Input: part model. Units: mm. Frame: model coordinates. Face numbers are marked on the shaded views. A direction names the side the tool comes from. Coordinates: 2 decimals unless noted, no trailing zeros. Loops run counter-clockwise (first coordinate to the right, second up) from the corner with the lowest first, then second, coordinate; pieces in that order, holes last. Notation, with made-up numbers: (68.5, 32.25) -> (91.5, 32.25) arc R25 ccw to (91.5, 46.25) -> close; hole circle Ø3 at (20.25, -31.5). An arc over 180 degrees is marked (long way). Put each result on its own line as item: value. Start each with the question number.
1) Contact query for flat-ended pins moving along their axis: P1, Ø10.5, axis at x = 27, z = 6, coming from the -Y side; P2, Ø3, axis at y = -16.5, z = 3, coming from the -X side; P3, Ø8.5, axis at x = 28.575, z = 5.715, coming from the -Y side. Output: stop coordinate, or through.
2) Pull-direction query (X, two-part tool) for the marked faces 4, 5 and 6; classes: pulls with the +X half, pulls with the -X half, needs draft (parallel to the pull), parting line crosses it, or undercut.
3) Cut plane C-C (y = -21.5). Return the cut outline in (x, z).
4) Cut plane B-B (y = -2). Return the cut outline in (x, z) (3 decimals).
5) Set-up query: the marked faces 1, 2 and 3. Return all of +Z, -Z, +X, -X, +Y, -Y with unobstructed straight access to the full face (end or side cutting, diameter ignored); none if empty.
6) Cut plane A-A (z = 0). Return the cut outline in (x, y).
7) Material intervals for L1, parallel to Y at x = 10.5, z = 6.5; L2, parallel to Y at x = 25.5, z = 10.5; L3, parallel to Z at x = 1, y = -10, sorted ascending.
from build123d import *

# Parameters (mm, degrees)
F0_R     = 2.9718
F0_R_2   = 7.1628
F0_R_3   = 1.9812
F0_R_4   = 4.7752
F1_DEPTH = 6.35
F2_DEPTH = 6.35
F3_DEPTH = 25.4


with BuildPart() as f1:
    # F0 (on Front) → F1 (new body)
    with BuildSketch(Plane.XZ):
        with BuildLine():
            Line((-2.766164, 5.258687), (-20.029118, 11.688779))
            ThreePointArc((-20.029118, 11.688779), (-25.125379, 9.358682), (-22.795282, 4.262421))
            Line((-22.795282, 4.262421), (-1.383082, -3.713179))
            ThreePointArc((-1.383082, -3.713179), (-0.694015, -3.901148), (0.017603, -3.962361))
            Line((0.017603, -3.962361), (28.617427, -3.835306))
            ThreePointArc((28.617427, -3.835306), (37.933712, 7.618851), (24.882816, 14.522833))
            Line((24.882816, 14.522833), (3.063727, 5.376418))
            ThreePointArc((3.063727, 5.376418), (0.160003, 4.76186), (-2.766164, 5.258687))
        make_face()
        Circle(F0_R, mode=Mode.SUBTRACT)
        with Locations((-21.4122, 7.9756)):
            Circle(F0_R, mode=Mode.SUBTRACT)
        with Locations((28.575, 5.715)):
            Circle(F0_R_2, mode=Mode.SUBTRACT)
        with Locations((-21.4122, 7.9756)):
            Circle(F0_R)
        with Locations((-21.4122, 7.9756)):
            Circle(F0_R_3, mode=Mode.SUBTRACT)
        with Locations((-21.4122, 7.9756)):
            Circle(F0_R_3)
        Circle(F0_R)
        Circle(F0_R_3, mode=Mode.SUBTRACT)
        Circle(F0_R_3)
        with Locations((28.575, 5.715)):
            Circle(F0_R_2)
        with Locations((28.575, 5.715)):
            Circle(F0_R_4, mode=Mode.SUBTRACT)
        with Locations((28.575, 5.715)):
            Circle(F0_R_4)
    extrude(amount=-F1_DEPTH)

    # F0 (on Front) → F2 (join)
    with BuildSketch(Plane.XZ):
        with Locations((-21.4122, 7.9756)):
            Circle(F0_R)
        with Locations((-21.4122, 7.9756)):
            Circle(F0_R_3, mode=Mode.SUBTRACT)
        Circle(F0_R)
        Circle(F0_R_3, mode=Mode.SUBTRACT)
        with Locations((28.575, 5.715)):
            Circle(F0_R_2)
        with Locations((28.575, 5.715)):
            Circle(F0_R_4, mode=Mode.SUBTRACT)
    extrude(amount=F2_DEPTH)

    # F0 (on Front) → F3 (join)
    with BuildSketch(Plane.XZ):
        with Locations((-21.4122, 7.9756)):
            Circle(F0_R_3)
        Circle(F0_R_3)
    extrude(amount=F3_DEPTH)


solid = f1.part
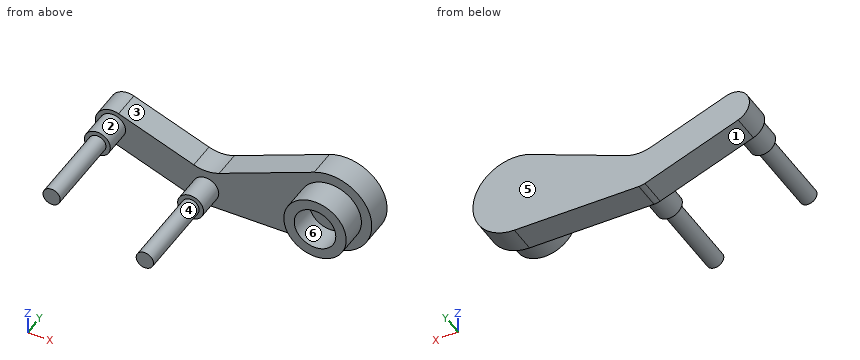
Results found:
1. P1: stops at y = -6.35
1. P2: stops at x = -1.29
1. P3: stops at y = 0
2. face 4: parting line crosses it
2. face 5: needs draft
2. face 6: undercut
3. outline: circle Ø3.96 at (-21.41, 7.98); circle Ø3.96 at (0, 0)
4. outline: circle Ø5.944 at (-21.412, 7.976); circle Ø5.944 at (0, 0); circle Ø14.326 at (28.575, 5.715); hole circle Ø9.55 at (28.575, 5.715)
5. face 1: -Z, -X, +Y, -Y
5. face 2: -Y
5. face 3: +Z, +Y, -Y
6. outline: (-11.35, 0) -> (-2.97, 0) -> (-2.97, -6.35) -> (-1.98, -6.35) -> (-1.98, -25.4) -> (1.98, -25.4) -> (1.98, -6.35) -> (2.97, -6.35) -> (2.97, 0) -> (24.26, 0) -> (24.26, -6.35) -> (32.89, -6.35) -> (32.89, 0) -> (36.23, 0) -> (36.23, 6.35) -> (-11.35, 6.35) -> close
7. L1: y = 0 to 6.35
7. L2: y = -6.35 to 6.35
7. L3: z = -1.71 to 1.71
